Read the model definition and answer for the solid it produces. Units are mm, in the model's axes. A direction names the side the tool comes from. Round coordinates to 2 decimals unless told otherwise and drop trailing zeros. Write each loop counter-clockwise with the first axis right and the second up, starting at its lowest first coordinate (ties: lowest second). Pieces come first, ordered by that corner, then holes. Notation, with made-up numbers: (68.5, -18.5) - (84.5, -18.5) arc R14 cw to (84.5, -10.5) - close; hole circle Ø7 at (-31, 73.25). An arc over 180 degrees is marked (long way). One line per item, written item: value. Start each with the question number.
(1) Find the intervals of material crossed by L1, parallel to Y at x = 0, z = 4.5 (3 decimals); L2, parallel to Y at x = 0, z = 2.5; L3, parallel to X at y = -1, z = 6.5, in increasing order.
(2) For faces 4 (the face through (-1.2, 0, 5)), 5 (the face through (-9.73, 8.92, 6.74)), 6 (the face through (0, -3, 9.35)), determine the directions among +Z, -Z, +X, -X, +Y, -Y from which every point of the face is accessible in a straight line to the end or side of a thin tool.
(3) A cutting plane is placed at B-B, the plane x = 0. Determine the outline of the cut face in (y, z) (3 decimals).
(4) Flat-ended cylindrical pins translate along their axes: pin 1 Ø4 at (y, z) = (-4.5, 1.5) entering from +X; pin 2 Ø5 at (y, z) = (8.5, 7) entering from +X; pin 3 Ø1 at (y, z) = (-10, 7) entering from -X; pin 4 Ø8 at (x, y) = (1.5, 6.5) entering from -Z. Find the tip coordinate at first contact, or state that the pin passes through.
(5) A cutting plane is placed at A-A, the plane y = 0. Determine the outline of the cut face in (x, z) (3 decimals), plus the area to 3 significant figures.
(6) The mould has two halves that part along Z. Classify faces 1 (the face through (-2.899, -13.057, 0.493)), 2 (the face through (0, -3, 0)), 3 (the face through (-9.73, 8.92, 2.57)): +Z half, -Z half, draft (parallel to the pull), parting line (faces both ways), or undercut.
(7) A cutting plane is placed at D-D, the plane y = 10. Determine the outline of the cut face in (x, z) (3 decimals).
(8) A cutting plane is placed at C-C, the plane z = 4.75. Determine the outline of the cut face in (x, y) (3 decimals), plus the area to 3 significant figures.
from build123d import *

# Parameters (mm, degrees)
SKETCH2_R           = 13.375
BOSS_EXTRUDE1_DEPTH = 1
SKETCH3_R           = 13.2
BOSS_EXTRUDE2_DEPTH = 3.175
SKETCH4_R           = 13.375
BOSS_EXTRUDE3_DEPTH = 1
SKETCH5_R           = 13.2
BOSS_EXTRUDE4_DEPTH = 3.175
SKETCH6_R           = 13.375
BOSS_EXTRUDE5_DEPTH = 1
CUT_EXTRUDE2_DEPTH  = 10.35


with BuildPart() as part:
    # Sketch2 → Boss-Extrude1 (new body)
    with BuildSketch(Plane.XY):
        Circle(SKETCH2_R)
    extrude(amount=BOSS_EXTRUDE1_DEPTH)

    # Sketch3 → Boss-Extrude2 (add)
    with BuildSketch(Plane.XY.offset(1)):
        Circle(SKETCH3_R)
    extrude(amount=BOSS_EXTRUDE2_DEPTH)

    # Sketch4 → Boss-Extrude3 (add)
    with BuildSketch(Plane.XY.offset(4.175)):
        Circle(SKETCH4_R)
    extrude(amount=BOSS_EXTRUDE3_DEPTH)

    # Sketch5 → Boss-Extrude4 (add)
    with BuildSketch(Plane.XY.offset(5.175)):
        Circle(SKETCH5_R)
    extrude(amount=BOSS_EXTRUDE4_DEPTH)

    # Sketch6 → Boss-Extrude5 (add)
    with BuildSketch(Plane.XY.offset(8.35)):
        Circle(SKETCH6_R)
    extrude(amount=BOSS_EXTRUDE5_DEPTH)

    # Sketch8 → Cut-Extrude2 (cut, through all)
    with BuildSketch(Plane(origin=(0, 0, 0), x_dir=(-1, 0, 0), z_dir=(0, 0, -1))):
        with BuildLine():
            Line((1.2, 1.132475165), (1.2, -1.132475165))
            ThreePointArc((1.2, -1.132475165), (-1.65, 0), (1.2, 1.132475165))
        make_face()
    extrude(amount=-CUT_EXTRUDE2_DEPTH, mode=Mode.SUBTRACT)


solid = part.part
Here are the results:
1. L1: -13.375 to -1.65, 1.65 to 13.375
1. L2: -13.2 to -1.65, 1.65 to 13.2
1. L3: -13.16 to -1.2, 1.31 to 13.16
2. face 4: +Z, -Z
2. face 5: none
2. face 6: +Z, +X, -X, +Y, -Y
3. outline: (-13.375, 0) - (-1.65, 0) - (-1.65, 9.35) - (-13.375, 9.35) - (-13.375, 8.35) - (-13.2, 8.35) - (-13.2, 5.175) - (-13.375, 5.175) - (-13.375, 4.175) - (-13.2, 4.175) - (-13.2, 1) - (-13.375, 1) - close; (1.65, 0) - (13.375, 0) - (13.375, 1) - (13.2, 1) - (13.2, 4.175) - (13.375, 4.175) - (13.375, 5.175) - (13.2, 5.175) - (13.2, 8.35) - (13.375, 8.35) - (13.375, 9.35) - (1.65, 9.35) - close
4. pin 1: x = 13.13
4. pin 2: x = 11.76
4. pin 3: x = -9.16
4. pin 4: z = 0
5. outline: (-13.375, 0) - (-1.2, 0) - (-1.2, 9.35) - (-13.375, 9.35) - (-13.375, 8.35) - (-13.2, 8.35) - (-13.2, 5.175) - (-13.375, 5.175) - (-13.375, 4.175) - (-13.2, 4.175) - (-13.2, 1) - (-13.375, 1) - close; (1.65, 0) - (13.375, 0) - (13.375, 1) - (13.2, 1) - (13.2, 4.175) - (13.375, 4.175) - (13.375, 5.175) - (13.2, 5.175) - (13.2, 8.35) - (13.375, 8.35) - (13.375, 9.35) - (1.65, 9.35) - close
5. area: 221 mm²
6. face 1: draft
6. face 2: -Z half
6. face 3: undercut
7. outline: (-8.882, 0) - (8.882, 0) - (8.882, 1) - (8.616, 1) - (8.616, 4.175) - (8.882, 4.175) - (8.882, 5.175) - (8.616, 5.175) - (8.616, 8.35) - (8.882, 8.35) - (8.882, 9.35) - (-8.882, 9.35) - (-8.882, 8.35) - (-8.616, 8.35) - (-8.616, 5.175) - (-8.882, 5.175) - (-8.882, 4.175) - (-8.616, 4.175) - (-8.616, 1) - (-8.882, 1) - close
8. outline: circle Ø26.75 at (0, 0); hole (-1.2, -1.132) arc R1.65 ccw (long way) to (-1.2, 1.132) - close
8. area: 554 mm²
